```python
from build123d import *

# Parameters (mm, degrees)
F0_W      = 200
F0_H      = 120
F1_DEPTH  = 5
F2_R      = 1.5
F2_W      = 20
F2_H      = 15
F3_DEPTH  = 25
F4_R      = 1.5
F5_DEPTH  = 5.001
F6_R      = 2
F7_DEPTH  = 5.001
F8_R      = 1.5
F9_DEPTH  = 5.001
F10_R     = 1.5
F11_DEPTH = 5.001
F12_R     = 1.5
F13_DEPTH = 5.001


with BuildPart() as f1:
    # F0 (on Top) → F1 (new body)
    with BuildSketch(Plane.XY):
        Rectangle(F0_W, F0_H)
    extrude(amount=F1_DEPTH)

    # F2 (on face) → F3 (cut)
    with BuildSketch(Plane.XY.offset(5)):
        with Locations((-90, 52)):
            Circle(F2_R)
        with Locations((-52, 52)):
            Circle(F2_R)
        with Locations((-90, -52)):
            Circle(F2_R)
        with Locations((-52, -52)):
            Circle(F2_R)
        with Locations((-71, 25)):
            Rectangle(F2_W, F2_H)
        with Locations((-71, -25)):
            Rectangle(F2_W, F2_H)
    extrude(amount=-F3_DEPTH, mode=Mode.SUBTRACT)

    # F4 (on face) → F5 (cut, through all)
    with BuildSketch(Plane.XY.offset(5)):
        with Locations((26, -29)):
            Circle(F4_R)
        with Locations((26, 29)):
            Circle(F4_R)
        with Locations((75, -29)):
            Circle(F4_R)
        with Locations((75, 29)):
            Circle(F4_R)
    extrude(amount=-F5_DEPTH, mode=Mode.SUBTRACT)

    # F6 (on face) → F7 (cut, through all)
    with BuildSketch(Plane(origin=(0, 0, 0), x_dir=(1, 0, 0), z_dir=(0, 0, -1))):
        with Locations((85, 19.5)):
            Circle(F6_R)
        with Locations((85, -19.5)):
            Circle(F6_R)
    extrude(amount=-F7_DEPTH, mode=Mode.SUBTRACT)

    # F8 (on face) → F9 (cut, through all)
    with BuildSketch(Plane.XY.offset(5)):
        with Locations((-35, 44)):
            Circle(F8_R)
        with Locations((-35, 6.7)):
            Circle(F8_R)
        with Locations((2.3, 44)):
            Circle(F8_R)
        with Locations((2.3, 6.7)):
            Circle(F8_R)
    extrude(amount=-F9_DEPTH, mode=Mode.SUBTRACT)

    # F10 (on face) → F11 (cut, through all)
    with BuildSketch(Plane.XY.offset(5)):
        with Locations((-40, -21)):
            Circle(F10_R)
        with Locations((-40, -50)):
            Circle(F10_R)
        with Locations((9, -21)):
            Circle(F10_R)
        with Locations((9, -50)):
            Circle(F10_R)
    extrude(amount=-F11_DEPTH, mode=Mode.SUBTRACT)

    # F12 (on face) → F13 (cut, through all)
    with BuildSketch(Plane.XY.offset(5)):
        with Locations((-50, 34.5)):
            Circle(F12_R)
        with Locations((-50, -34.5)):
            Circle(F12_R)
    extrude(amount=-F13_DEPTH, mode=Mode.SUBTRACT)


solid = f1.part
```
Verification items for the finished model (mm, model axes). A direction names the side the tool comes from. Round coordinates to 2 decimals unless told otherwise and drop trailing zeros. Write each loop counter-clockwise with the first axis right and the second up, starting at its lowest first coordinate (ties: lowest second). Pieces come first, ordered by that corner, then holes. Notation, with made-up numbers: (-2, -38) -> (11, -38) arc R12 cw to (11, -25) -> close; hole circle Ø4 at (-23, 67). An arc over 180 degrees is marked (long way). Write each question's results on one line, items separated by ' | '.
Q1. Thickness scan on probe 1 along Y at (x, z) = (9, 1.5); probe 2 along X at (y, z) = (19.5, 1.15); probe 3 along Y at (x, z) = (2.3, 1.1). Record the ranges inside material, lowest first.
Derived:
probe 1: y = -60 to -51.5, -48.5 to -22.5, -19.5 to 60 | probe 2: x = -100 to -81, -61 to 83, 87 to 100 | probe 3: y = -60 to 5.2, 8.2 to 42.5, 45.5 to 60
Q2. Draft check along X on faces 3 (the face through (-1, 60, 2)), 4 (the face through (-71, -17.5, 3)), 5 (the face through (100, -1, 2)). Enter one of: released by +X, released by -X, zero draft, split by the parting line, or undercut.
Derived:
face 3: zero draft | face 4: undercut | face 5: released by +X
Q3. Sectioned sample at A-A, the plane z = 3.1. Give the number of separate pieces and of enclosed holes in the cut face, and give its area (3 significant figures).
Derived:
separate pieces: 1 | enclosed holes: 22 | area: 23,200 mm²
Q4. Go/stop test with a flat-tipped pin: pin 1 Ø3.5 at (x, y) = (85, 19.5) entering from -Z. Record where the tip stops, or that it passes through.
Derived:
pin 1: passes through
Q5. Access from +Z, -Z, +X, -X, +Y, -Y to the whole of each face (thin tool, end or side, straight path). Record for faces 1 (the face through (-71, -32.5, 3)), 2 (the face through (-100, -1, 2)).
Derived:
face 1: +Z, -Z | face 2: +Z, -Z, -X, +Y, -Y
Q6. Sectioned sample at B-B, the plane x = -77.5. Record the boundary of the cut face in (y, z), and give its area (3 significant figures).
Derived:
outline: (-60, 0) -> (-32.5, 0) -> (-32.5, 5) -> (-60, 5) -> close; (-17.5, 0) -> (17.5, 0) -> (17.5, 5) -> (-17.5, 5) -> close; (32.5, 0) -> (60, 0) -> (60, 5) -> (32.5, 5) -> close | area: 450 mm²
